Autodesk Inventor part; units mm, degrees
ref_plane "YZ Plane" through (0, 0, 0) normal (1, 0, 0) x (0, 1, 0)
ref_plane "XZ Plane" through (0, 0, 0) normal (0, 1, 0) x (-1, 0, 0)
ref_plane "XY Plane" through (0, 0, 0) normal (0, 0, 1) x (1, 0, 0)
sketch "Sketch1" plane through (0, 0, 0) normal (1, 0, 0) x (0, 1, 0)
  point P0 (0, 0)
sketch "Sketch2" plane through (0, 0, 0) normal (1, 0, 0) x (0, 1, 0)
  circle A0 centre (0, 0) radius 6
  dimension "d0" = 12
extrude "Extrusion1" add sketch "Sketch2" along normal blind 80
sketch "Sketch3" plane through (0, 0, 0) normal (-1, 0, 0) x (0, 0, 1)
  circle A0 centre (0, 0) radius 3.25
  dimension "d3" = 6.5
extrude "Extrusion2" add sketch "Sketch3" along normal blind 5
fillet "Fillet1" radius 1 1 edges at (0, -6, 0)
fillet "Fillet2" radius 1 1 edges at (80, -6, 0)
properties part number "Handle_holder"
Work out the finished part from the listing and answer in its coordinate system (mm). A direction names the side the tool comes from. Coordinates: 2 decimals unless noted, no trailing zeros. Order: outer loops, then holes, each group sorted by start corner. A loop starts at its lowest first (then second) coordinate and runs counter-clockwise, first axis right, second up. Notation, with made-up numbers: M 41.25,-14.5 L 53.25,-14.5 A7 ccw 53.25,-4.5 Z; hole C 70.25,12.5 d10. An arc over 180 degrees is marked long. Use CSV: the item, a comma, the result in double quotes.
1) Section C-C on x = 38 is taken. Write down the section's boundary in (y, z).
Worked out:
outline,"C 0,0 d12"
2) Consider line 1 (X direction, y = -2.75, z = 2.75); line 2 (Y direction, x = 21, z = 2); line 3 (Y direction, x = 35.5, z = -5.25). Determine where each line is inside the solid, lowest interval first. Write a range as [from, to].
Worked out:
line 1,"x = [0, 80]"
line 2,"y = [-5.66, 5.66]"
line 3,"y = [-2.9, 2.9]"
3) Section A-A on y = 0 is taken. Write down the section's boundary in (x, z), plus the area to 3 significant figures.
Worked out:
outline,"M -5,-3.25 L 0,-3.25 L 0,-5 A1 ccw 1,-6 L 79,-6 A1 ccw 80,-5 L 80,5 A1 ccw 79,6 L 1,6 A1 ccw 0,5 L 0,3.25 L -5,3.25 Z"
area,"992 mm^2"
4) Flat-ended cylindrical pins translate along their axes: pin 1 Ø1 at (x, y) = (66.5, 5) entering from +Z; pin 2 Ø3 at (x, z) = (59, 3.5) entering from -Y; pin 3 Ø1 at (y, z) = (-0.5, 4.5) entering from -X. Find the tip coordinate at first contact, or state that the pin passes through.
Worked out:
pin 1,"stops at z = 3.97"
pin 2,"stops at y = -5.66"
pin 3,"stops at x = 0"
5) For faces 1 (the face through (-2.465, 1.978, -2.579)), 2 (the face through (-5, 0, 0)), determine the directions among +Z, -Z, +X, -X, +Y, -Y from which every point of the face is accessible in a straight line to the end or side of a thin tool.
Worked out:
face 1,"-X"
face 2,"+Z, -Z, -X, +Y, -Y"
